The model under review builds one solid part; all positions refer to its coordinate system, in mm. Coordinates: 2 decimals unless noted, no trailing zeros. Write each loop counter-clockwise with the first axis right and the second up, starting at its lowest first coordinate (ties: lowest second). Pieces come first, ordered by that corner, then holes. Notation, with made-up numbers: (11, -31.5) - (40, -31.5) arc R26 ccw to (40, -14.5) - close; hole circle Ø2 at (19.25, 16). An arc over 180 degrees is marked (long way). Put each result on its own line as item: value.
from build123d import *

# Parameters (mm, degrees)
F0_R     = 44.48852
F1_DEPTH = 9.5
F2_R     = 25.811478
F4_DEPTH = 8.7
F5_R     = 25.87177
F6_DEPTH = 25


with BuildPart() as f1:
    # F0 (on Front) → F1 (new body)
    with BuildSketch(Plane.XZ):
        Circle(F0_R)
    extrude(amount=-F1_DEPTH)

    # F2 (on Front) → F4 (join)
    with BuildSketch(Plane.XZ):
        Circle(F2_R)
    extrude(amount=-F4_DEPTH)

    # F5 (on Front) → F6 (cut)
    with BuildSketch(Plane.XZ):
        Circle(F5_R)
    extrude(amount=-F6_DEPTH, mode=Mode.SUBTRACT)


solid = f1.part
1. The part is to be moulded in two halves that separate along X. For faces 1 (the flat face through (19, 0, -19)), 2 (the cylindrical face through (-5.608, 4.684, -25.257)), 3 (the cylindrical face through (-9.64, 4.68, -43.43)), say which applies: +X half, -X half, draft (parallel to the pull), parting line (faces both ways), or undercut.
Determined:
face 1: draft
face 2: undercut
face 3: parting line
2. Consider section C-C on y = 7. State the section outline as (x, z) points.
Determined:
outline: circle Ø88.98 at (0, 0); hole circle Ø51.74 at (0, 0)
3. Consider section D-D on z = -35. State the section outline as (x, y) points, plus the area to 3 significant figures.
Determined:
outline: (-27.46, 0) - (27.46, 0) - (27.46, 9.5) - (-27.46, 9.5) - close
area: 522 mm^2
4. Consider section B-B on z = 0. State the section outline as (x, y) points, plus the area to 3 significant figures.
Determined:
outline: (-44.49, 0) - (-25.87, 0) - (-25.87, 9.5) - (-44.49, 9.5) - close; (25.87, 0) - (44.49, 0) - (44.49, 9.5) - (25.87, 9.5) - close
area: 354 mm^2
5. To check wall thickness, follow probe 1 along Z at (x, y) = (0, 6.75); probe 2 along X at (y, z) = (7.75, -13.5); probe 3 along Z at (x, y) = (5, 1.75). State the ranges of each line that lie inside material, in increasing order.
Determined:
probe 1: z = -44.49 to -25.87, 25.87 to 44.49
probe 2: x = -42.39 to -22.07, 22.07 to 42.39
probe 3: z = -44.21 to -25.38, 25.38 to 44.21
6. Consider section A-A on x = 0. State the section outline as (y, z) points, plus the area to 3 significant figures.
Determined:
outline: (0, -44.49) - (9.5, -44.49) - (9.5, -25.87) - (0, -25.87) - close; (0, 25.87) - (9.5, 25.87) - (9.5, 44.49) - (0, 44.49) - close
area: 354 mm^2
7. For pin 1 Ø3 at (y, z) = (2, 29.5) entering from +X; pin 2 Ø3 at (x, y) = (18, 2) entering from +Z; pin 3 Ø2 at (x, y) = (14.5, 6) entering from -Z; pin 4 Ø6 at (x, z) = (23.5, 7) entering from -Y, all flat-tipped, find the tip position at first contact; note any pin that passes through.
Determined:
pin 1: stops at x = 34.57
pin 2: stops at z = 41.32
pin 3: stops at z = -42.39
pin 4: stops at y = 0
